```python
from build123d import *

# Parameters (mm, degrees)
SKETCH1_W           = 130
SKETCH1_H           = 120
BOSS_EXTRUDE1_DEPTH = 3
CUT_EXTRUDE1_START  = -4
SKETCH2_W           = 20
SKETCH2_H           = 95
CUT_EXTRUDE1_DEPTH  = 5
CUT_EXTRUDE2_START  = -4
SKETCH3_R           = 1.6
CUT_EXTRUDE2_DEPTH  = 5


with BuildPart() as part:
    # Sketch1 → Boss-Extrude1 (new body)
    with BuildSketch(Plane(origin=(0, 0, 0), x_dir=(1, 0, 0), z_dir=(0, 1, 0))):
        Rectangle(SKETCH1_W, SKETCH1_H)
    extrude(amount=BOSS_EXTRUDE1_DEPTH)

    # Sketch2 → Cut-Extrude1 (cut)
    with BuildSketch(Plane(origin=(0, 3, 0), x_dir=(1, 0, 0), z_dir=(0, 1, 0)).offset(CUT_EXTRUDE1_START)):
        with Locations((-16.25, 0)):
            Rectangle(SKETCH2_W, SKETCH2_H)
    cut_extrude1 = extrude(amount=CUT_EXTRUDE1_DEPTH, mode=Mode.SUBTRACT)

    # Mirror1: Cut-Extrude1 across plane
    add(cut_extrude1.mirror(Plane(origin=(0, 0, 0), x_dir=(0, 0, 1), z_dir=(1, 0, 0))), mode=Mode.SUBTRACT)

    # Sketch3 → Cut-Extrude2 (cut)
    with BuildSketch(Plane(origin=(0, 3, 0), x_dir=(1, 0, 0), z_dir=(0, 1, 0)).offset(CUT_EXTRUDE2_START)):
        with Locations((44.5, 0)):
            Circle(SKETCH3_R)
    cut_extrude2 = extrude(amount=CUT_EXTRUDE2_DEPTH, mode=Mode.SUBTRACT)

    # Mirror2: Cut-Extrude2 across plane
    add(cut_extrude2.mirror(Plane(origin=(0, 0, 0), x_dir=(0, 0, 1), z_dir=(1, 0, 0))), mode=Mode.SUBTRACT)


solid = part.part
```
CAD build for the part. Positions are in the model's coordinates, mm. A direction names the side the tool comes from. Coordinates: 2 decimals unless noted, no trailing zeros. Order: outer loops, then holes, each group sorted by start corner. A loop starts at its lowest first (then second) coordinate and runs counter-clockwise, first axis right, second up. Notation, with made-up numbers: (-35, -23) - (16, -23) arc R15 ccw to (16, -12) - close; hole circle Ø7 at (46, 65.5). An arc over 180 degrees is marked (long way). Answer in a Markdown table with one row per item.
1. Slice it at A-A, the plane x = 44.5. List the corners of the cut face in (y, z), then the cut area to 3 significant figures.
Answer:
| item | result |
|---|---|
| outline | (0, -60) - (3, -60) - (3, -1.6) - (0, -1.6) - close; (0, 1.6) - (3, 1.6) - (3, 60) - (0, 60) - close |
| area | 350 mm² |
2. 3-axis set-ups, long thin cutter, end or side, ignore diameter. For faces 1 (the face through (-1, 1, -60)), 2 (the face through (16, 1, 47.5)): which of +Z, -Z, +X, -X, +Y, -Y reach the whole face in a straight line?
Answer:
| item | result |
|---|---|
| face 1 | -Z, +X, -X, +Y, -Y |
| face 2 | +Y, -Y |
3. Drill centre lines: L1, parallel to X at y = 0.45, z = 20.5; L2, parallel to Z at x = 10, y = 1.7; L3, parallel to Z at x = -44.5, y = 1.1. Where is each one in solid material? Low to high. Write a range as from..to.
Answer:
| item | result |
|---|---|
| L1 | -65..-26.25, -6.25..6.25, 26.25..65 |
| L2 | -60..-47.5, 47.5..60 |
| L3 | -60..-1.6, 1.6..60 |
4. Slice it at B-B, the plane z = 12. List the corners of the cut face in (x, y), then the cut area to 3 significant figures.
Answer:
| item | result |
|---|---|
| outline | (-65, 0) - (-26.25, 0) - (-26.25, 3) - (-65, 3) - close; (-6.25, 0) - (6.25, 0) - (6.25, 3) - (-6.25, 3) - close; (26.25, 0) - (65, 0) - (65, 3) - (26.25, 3) - close |
| area | 270 mm² |
5. Flat gauge pin, fed straight in: P1, Ø2.5, axis at x = 44.5, z = 0, coming from the -Y side. Where does the tip first touch, or does it go through?
Answer:
| item | result |
|---|---|
| P1 | through |
6. Slice it at D-D, the plane y = 1.65. List the corners of the cut face in (x, z), then the cut area to 3 significant figures.
Answer:
| item | result |
|---|---|
| outline | (-65, -60) - (65, -60) - (65, 60) - (-65, 60) - close; hole circle Ø3.2 at (-44.5, 0); hole (-26.25, -47.5) - (-6.25, -47.5) - (-6.25, 47.5) - (-26.25, 47.5) - close; hole (6.25, -47.5) - (26.25, -47.5) - (26.25, 47.5) - (6.25, 47.5) - close; hole circle Ø3.2 at (44.5, 0) |
| area | 11,800 mm² |
7. Pull direction X, two halves, no side cores. Call faces 3 (the face through (-65, 1, 1)), 4 (the face through (6.25, 1, 1)), 5 (the face through (-1, 1, 60)): +X half, -X half, draft (parallel to the pull), parting line (faces both ways), or undercut.
Answer:
| item | result |
|---|---|
| face 3 | -X half |
| face 4 | undercut |
| face 5 | draft |
8. Slice it at C-C, the plane z = 0. List the corners of the cut face in (x, y), then the cut area to 3 significant figures.
Answer:
| item | result |
|---|---|
| outline | (-65, 0) - (-46.1, 0) - (-46.1, 3) - (-65, 3) - close; (-42.9, 0) - (-26.25, 0) - (-26.25, 3) - (-42.9, 3) - close; (-6.25, 0) - (6.25, 0) - (6.25, 3) - (-6.25, 3) - close; (26.25, 0) - (42.9, 0) - (42.9, 3) - (26.25, 3) - close; (46.1, 0) - (65, 0) - (65, 3) - (46.1, 3) - close |
| area | 251 mm² |
